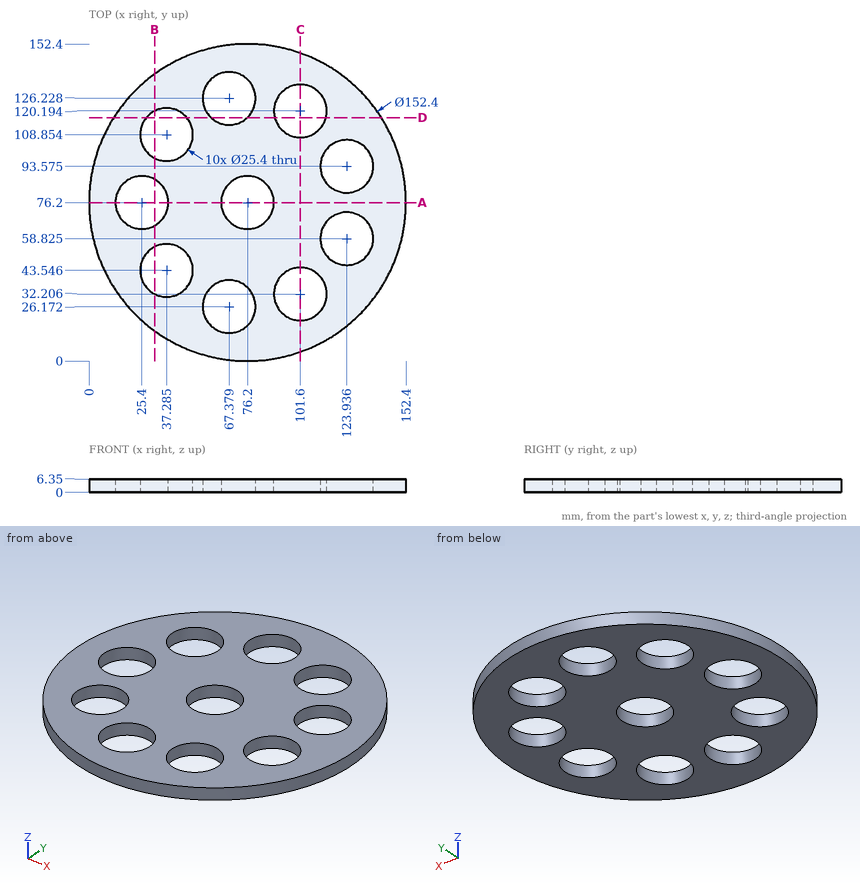
Design review of the part shown in the three views and the two pictorial views. Dimensions are in mm from the part's minimum x, y and z. Round coordinates to 2 decimals unless told otherwise and drop trailing zeros. Order: outer loops, then holes, each group sorted by start corner. A loop starts at its lowest first (then second) coordinate and runs counter-clockwise, first axis right, second up. Notation, with made-up numbers: (58.25, -13.75) - (67.25, -13.75) arc R17 ccw to (67.25, 9.25) - close; hole circle Ø10 at (-24, 68). An arc over 180 degrees is marked (long way). One line per question, with ' | ' between items.
Item 1: Take a section at C-C, the plane x = 101.6. Write out the cut boundary in (y, z), then the cut area to 3 significant figures.
Checks:
outline: (4.36, 0) - (19.51, 0) - (19.51, 6.35) - (4.36, 6.35) - close; (44.91, 0) - (107.49, 0) - (107.49, 6.35) - (44.91, 6.35) - close; (132.89, 0) - (148.04, 0) - (148.04, 6.35) - (132.89, 6.35) - close | area: 590 mm²
Item 2: For P1, Ø3, axis at y = 55, z = 3, coming from the -X side; P2, Ø2, axis at x = 120, z = 5.5, coming from the -Y side (1 decimal), all flat-tipped, find the tip position at first contact; note any pin that passes through.
Checks:
P1: x = 2.59 | P2: y = 13.2
Item 3: Take a section at B-B, the plane x = 31.5. Write out the cut boundary in (y, z).
Checks:
outline: (14.49, 0) - (32.24, 0) - (32.24, 6.35) - (14.49, 6.35) - close; (54.85, 0) - (65.06, 0) - (65.06, 6.35) - (54.85, 6.35) - close; (87.34, 0) - (97.55, 0) - (97.55, 6.35) - (87.34, 6.35) - close; (120.16, 0) - (137.91, 0) - (137.91, 6.35) - (120.16, 6.35) - close
Item 4: Take a section at D-D, the plane y = 117. Write out the cut boundary in (x, z).
Checks:
outline: (11.84, 0) - (27.54, 0) - (27.54, 6.35) - (11.84, 6.35) - close; (47.03, 0) - (58.65, 0) - (58.65, 6.35) - (47.03, 6.35) - close; (76.1, 0) - (89.31, 0) - (89.31, 6.35) - (76.1, 6.35) - close; (113.89, 0) - (140.56, 0) - (140.56, 6.35) - (113.89, 6.35) - close
Item 5: Wall thickness on line 1 (Y direction, x = 115, z = 5.5); line 2 (Y direction, x = 46, z = 2.75) (1 decimal); line 3 (Y direction, x = 33, z = 4) (1 decimal): over which ranges is each line inside the solid? List them lowest first. Write a range as [from, to].
Checks:
line 1: [10.62, 49.8], [67.85, 84.55], [102.6, 141.78] | line 2: [6.2, 34.3], [52.8, 99.6], [118.1, 146.2] | line 3: [13.4, 31.6], [55.5, 66], [86.4, 96.9], [120.8, 139]
Item 6: Take a section at A-A, the plane y = 76.2. Write out the cut boundary in (x, z), then the cut area to 3 significant figures.
Checks:
outline: (0, 0) - (12.7, 0) - (12.7, 6.35) - (0, 6.35) - close; (38.1, 0) - (63.5, 0) - (63.5, 6.35) - (38.1, 6.35) - close; (88.9, 0) - (152.4, 0) - (152.4, 6.35) - (88.9, 6.35) - close | area: 645 mm²
